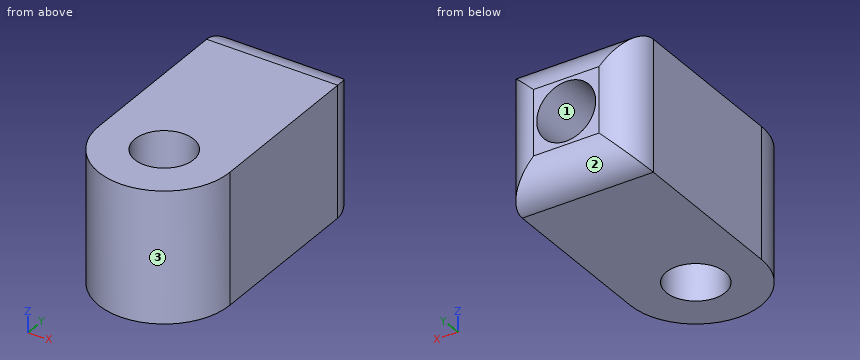
```python
from build123d import *

# Parameters (mm, degrees)
F0_R     = 0.9
F1_DEPTH = 4
F2_R     = 0.9
F3_DEPTH = 4.7
F4_R     = 1


with BuildPart() as f1:
    # F0 (on Top) → F1 (new body)
    with BuildSketch(Plane.XY):
        with BuildLine():
            Line((-136.606078, -64.349075), (-136.606078, -70.349075))
            ThreePointArc((-136.606078, -70.349075), (-134.606078, -72.349075), (-132.606078, -70.349075))
            Line((-132.606078, -70.349075), (-132.606078, -64.349075))
            Line((-132.606078, -64.349075), (-136.606078, -64.349075))
        make_face()
        with Locations((-134.606078, -70.349075)):
            Circle(F0_R, mode=Mode.SUBTRACT)
    extrude(amount=F1_DEPTH)

    # F2 (on face) → F3 (cut)
    with BuildSketch(Plane(origin=(0, -64.349075, 0), x_dir=(-1, 0, 0), z_dir=(0, 1, 0))):
        with Locations((134.606078, 2)):
            Circle(F2_R)
    extrude(amount=-F3_DEPTH, mode=Mode.SUBTRACT)

    # F4
    f4_edges = [f1.edges().sort_by_distance(p)[0] for p in [
        (-132.606078, -64.349075, 2),
        (-134.606078, -64.349075, 0),
        (-136.606078, -64.349075, 2),
        (-134.606078, -64.349075, 4),
    ]]
    fillet(f4_edges, radius=F4_R)


solid = f1.part
```
Build history of the part. All positions in model axes, mm. Face numbers are marked on the shaded views. Give positions to 0.01 mm unless a question says otherwise; leave off trailing zeros. Loops run counter-clockwise (first coordinate to the right, second up) from the corner with the lowest first, then second, coordinate; pieces in that order, holes last. Notation, with made-up numbers: (-5, 26.25) -> (32, 26.25) arc R21 cw to (32, 35.25) -> close; hole circle Ø8 at (-30, 10). An arc over 180 degrees is marked (long way). One line per question, with ' | ' between items. Start each with the question number.
1) Cut at D-D (x = -134.7). Give the cut face in (y, z).
2) Two-plate mould, pull along X, no slides. Class the marked faces 1, 2 and 3: released by +X, released by -X, zero draft, split by the parting line, or undercut.
3) Probe L1, parallel to X at y = -67.5, z = 1.6; L2, parallel to X at y = -68.25, z = 2.6; L3, parallel to Y at x = -134.05, z = 3.3. List the from-to ranges inside material, lowest first.
4) Pin check, flat tip, straight feed: pin 1 (0.5 mm diameter, centred on x = -135, z = 2, fed in from +Y). Stop position of the tip, or through.
5) Cut at A-A (x = -134.1). Give the cut face in (y, z), plus the area to 3 significant figures.
6) Cut at B-B (z = 2). Give the cut face in (x, y), plus the area to 3 significant figures.
7) Cut at C-C (y = -70). Give the cut face in (x, z).
Return value:
1) outline: (-72.35, 0) -> (-71.24, 0) -> (-71.24, 4) -> (-72.35, 4) -> close; (-69.45, 0) -> (-65.35, 0) arc R1 ccw to (-64.35, 1) -> (-64.35, 1.1) -> (-69.05, 1.1) -> (-69.05, 2.9) -> (-64.35, 2.9) -> (-64.35, 3) arc R1 ccw to (-65.35, 4) -> (-69.45, 4) -> close
2) face 1: undercut | face 2: zero draft | face 3: split by the parting line
3) L1: -136.61 to -135.41, -133.8 to -132.61 | L2: -136.61 to -135.28, -133.94 to -132.61 | L3: -72.27 to -71.06, -69.64 to -64.4
4) pin 1: y = -69.05
5) outline: (-72.28, 0) -> (-71.09, 0) -> (-71.09, 4) -> (-72.28, 4) -> close; (-69.6, 0) -> (-65.35, 0) arc R1 ccw to (-64.35, 1) -> (-64.35, 1.26) -> (-69.05, 1.26) -> (-69.05, 2.74) -> (-64.35, 2.74) -> (-64.35, 3) arc R1 ccw to (-65.35, 4) -> (-69.6, 4) -> close | area: 18.4 mm^2
6) outline: (-136.61, -70.35) arc R2 ccw to (-132.61, -70.35) -> (-132.61, -65.35) arc R1 ccw to (-133.61, -64.35) -> (-133.71, -64.35) -> (-133.71, -69.05) -> (-135.51, -69.05) -> (-135.51, -64.35) -> (-135.61, -64.35) arc R1 ccw to (-136.61, -65.35) -> close; hole circle Ø1.8 at (-134.61, -70.35) | area: 18.8 mm^2
7) outline: (-136.61, 0) -> (-135.44, 0) -> (-135.44, 4) -> (-136.61, 4) -> close; (-133.78, 0) -> (-132.61, 0) -> (-132.61, 4) -> (-133.78, 4) -> close
